The figure shows three views and two pictorial views of one solid part (mm, origin at its lowest corner). Answer the questions. Round coordinates to 2 decimals unless told otherwise and drop trailing zeros. Write each loop counter-clockwise with the first axis right and the second up, starting at its lowest first coordinate (ties: lowest second). Pieces come first, ordered by that corner, then holes. Notation, with made-up numbers: (-25.75, 88.5) -> (-11.75, 88.5) arc R7 cw to (-11.75, 96.5) -> close; hole circle Ø2 at (73.5, 49.5). An arc over 180 degrees is marked (long way). One line per item, written item: value.
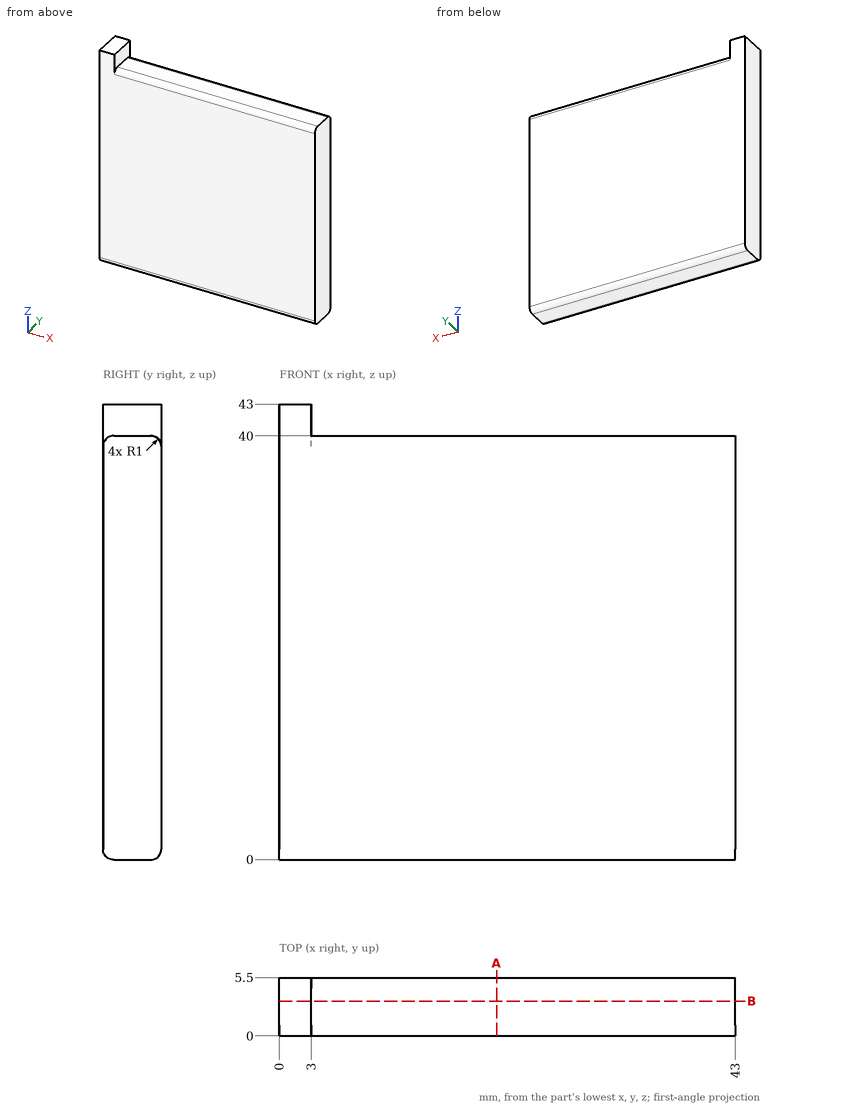
(1) Consider probe 1 along Z at (x, y) = (24, 2); probe 2 along Z at (x, y) = (15, 0.5). Determine where each line is inside the solid, lowest interval first.
Reported:
probe 1: z = 0 to 40
probe 2: z = 0.13 to 39.87
(2) Find section A-A on x = 20.5. Give the vertices of the cut face in (y, z), plus the area to 3 significant figures.
Reported:
outline: (0, 1) arc R1 ccw to (1, 0) -> (4.5, 0) arc R1 ccw to (5.5, 1) -> (5.5, 39) arc R1 ccw to (4.5, 40) -> (1, 40) arc R1 ccw to (0, 39) -> close
area: 219 mm2
(3) Flat-ended cylindrical pins translate along their axes: pin 1 Ø1 at (x, y) = (25.5, 4) entering from +Z; pin 2 Ø1.2 at (y, z) = (2.5, 41) entering from +X. Find the tip coordinate at first contact, or state that the pin passes through.
Reported:
pin 1: stops at z = 40
pin 2: stops at x = 3
(4) Find section B-B on y = 3.3. Give the vertices of the cut face in (x, z).
Reported:
outline: (0, 0) -> (43, 0) -> (43, 40) -> (3, 40) -> (3, 43) -> (0, 43) -> close
